Autodesk Inventor part; units mm, degrees
ref_plane "Work Plane2" through (7.15, 0, -16.233) normal (1, 0, 0) x (0, 0, -1)
ref_plane "Work Plane3" through (7.15, 0, -2.05) normal (1, 0, 0) x (0, 0, -1)
ref_plane "YZ Plane" through (0, 0, 0) normal (1, 0, 0) x (0, 1, 0)
sketch "Sketch1" plane through (0, 0, 0) normal (0, 1, 0) x (-1, 0, 0)
  line L0 (0, 0) -> (22.85, 0)
  line L1 (22.85, 0) -> (22.85, -100)
  line L2 (22.85, -100) -> (0, -100)
  line L3 (0, -100) -> (0, 0)
  circle A0 centre (7.12, -92.8) radius 4
  circle A1 centre (7.12, -64.4) radius 4
  circle A2 centre (7.12, -35.95) radius 4
  circle A3 centre (7.12, -7.71) radius 4
  circle A4 centre (7.12, -21.73) radius 1.5
  circle A5 centre (7.12, -49.67) radius 1.5
  circle A6 centre (7.12, -78.83) radius 1.5
  line L4 (7.12, -7.71) -> (-9.9799, -7.71) construction
  line L5 (7.12, -35.95) -> (-7.15, -35.95) construction
  line L6 (7.12, -64.4) -> (-7.15, -64.4) construction
  line L7 (7.12, -92.8) -> (-7.15, -92.8) construction
  line L8 (0, -27.427) -> (-7.15, -27.427)
  line L9 (0, -44.473) -> (-7.15, -44.473)
  line L10 (0, -55.877) -> (-7.15, -55.877)
  line L11 (0, -72.923) -> (-7.15, -72.923)
  line L12 (0, -84.277) -> (-7.15, -84.277)
  line L13 (0, -98.46) -> (-7.15, -98.46)
  line L14 (0, -2.05) -> (-7.15, -2.05)
  line L15 (0, -16.233) -> (-7.15, -16.233)
  line L16 (-7.15, -2.05) -> (-7.15, -16.233)
  line L17 (-7.15, -27.427) -> (-7.15, -44.473)
  line L18 (-7.15, -55.877) -> (-7.15, -72.923)
  line L19 (-7.15, -84.277) -> (-7.15, -98.46)
  line L20 (-7.15, 0) -> (-7.15, -100) construction
  dimension "d0" = 22.85
  dimension "d1" = 100
  dimension "d2" = 8
  dimension "d3" = 8
  dimension "d4" = 8
  dimension "d5" = 8
  dimension "d7" = 0
  dimension "d8" = 0
  dimension "d9" = 0
  dimension "d10" = 7.71
  dimension "d11" = 35.95
  dimension "d12" = 64.4
  dimension "d13" = 92.8
  dimension "d14" = 3
  dimension "d15" = 3
  dimension "d16" = 3
  dimension "d17" = 7.12
  dimension "d18" = 7.12
  dimension "d19" = 0
  dimension "d20" = 0
  dimension "d21" = 21.73
  dimension "d22" = 49.67
  dimension "d23" = 78.83
  dimension "d28" = 8.523
  dimension "d29" = 8.523
  dimension "d30" = 8.523
  dimension "d31" = 8.523
  dimension "d32" = 8.523
  dimension "d33" = 5.66
  dimension "d34" = 5.66
  dimension "d35" = 8.523
  dimension "d36" = 100
  dimension "d42" = 7.15
extrude "Extrusion1" add sketch "Sketch1" against normal blind 3
ref_plane "Work Plane2" through (7.15, 0, -16.233) normal (1, 0, 0) x (0, 0, -1)
ref_plane "Work Plane3" through (7.15, 0, -2.05) normal (1, 0, 0) x (0, 0, -1)
sketch "Sketch3" plane through (7.15, 0, -2.05) normal (1, 0, 0) x (0, 0, -1)
  line L0 (0, 0) -> (14.183, 0)
  line L1 (14.183, -3) -> (0, -3)
  line L2 (14.183, 0) -> (14.183, -3)
  line L3 (0, 0) -> (0, -3)
  line L4 (25.377, 0) -> (42.423, 0)
  line L5 (25.377, 0) -> (25.377, -3)
  line L6 (42.423, -3) -> (25.377, -3)
  line L7 (42.423, 0) -> (42.423, -3)
  line L8 (53.827, 0) -> (70.873, 0)
  line L9 (53.827, 0) -> (53.827, -3)
  line L10 (70.873, -3) -> (53.827, -3)
  line L11 (70.873, 0) -> (70.873, -3)
  line L12 (82.227, 0) -> (96.41, 0)
  line L13 (82.227, 0) -> (82.227, -3)
  line L14 (96.41, -3) -> (82.227, -3)
  line L15 (96.41, 0) -> (96.41, -3)
  line L16 (0, 0) -> (0, -40)
  line L17 (0, -40) -> (5.4, -40)
  line L18 (14.183, 0) -> (14.183, -20)
  line L19 (5.4, -40) -> (5.4, -28.783)
  line L20 (14.183, -20) -> (5.4, -28.783)
  line L21 (96.41, 0) -> (96.41, -40)
  line L22 (96.41, -40) -> (91.01, -40)
  line L23 (82.227, 0) -> (82.227, -20)
  line L24 (91.01, -40) -> (91.01, -28.783)
  line L25 (82.227, -20) -> (91.01, -28.783)
  line L26 (70.873, 0) -> (70.873, -20)
  line L27 (53.827, 0) -> (53.827, -20)
  line L28 (70.873, -20) -> (65.05, -25.823)
  line L29 (65.05, -25.823) -> (65.05, -40)
  line L30 (65.05, -40) -> (59.65, -40)
  line L31 (59.65, -40) -> (59.65, -25.823)
  line L32 (59.65, -25.823) -> (53.827, -20)
  line L33 (62.35, -40) -> (62.35, 0) construction
  line L34 (53.827, 0) -> (70.873, 0)
  line L35 (42.423, 0) -> (42.423, -20)
  line L36 (25.377, 0) -> (25.377, -20)
  line L37 (42.423, -20) -> (36.6, -25.823)
  line L38 (36.6, -25.823) -> (36.6, -40)
  line L39 (36.6, -40) -> (31.2, -40)
  line L40 (31.2, -40) -> (31.2, -25.823)
  line L41 (31.2, -25.823) -> (25.377, -20)
  line L42 (33.9, -40) -> (33.9, 0) construction
  point P0 (82.227, -3)
  dimension "d46" = 40
  dimension "d47" = 5.4
  dimension "d48" = 20
  dimension "d51" = 135
  dimension "d56" = 135
  dimension "d57" = 5.4
  dimension "d58" = 40
  dimension "d59" = 20
  dimension "d61" = 20
  dimension "d62" = 135
  dimension "d63" = 135
  dimension "d64" = 5.4
  dimension "d66" = 20
  dimension "d67" = 20
  dimension "d68" = 135
  dimension "d69" = 135
  dimension "d70" = 5.4
  dimension "d71" = 20
extrude "Extrusion2" add sketch "Sketch3" against normal blind 3
fillet "Fillet1" radius 4 4 edges at (7.15, 0, -9.1415) (7.15, 0, -35.95) (7.15, 0, -64.4) (7.15, 0, -91.3685)
chamfer "Chamfer1" distance 4 angle 45 4 edges at (4.15, -3, -9.1415) (4.15, -3, -35.95) (4.15, -3, -64.4) (4.15, -3, -91.3685)
equation "\"d18\" = d17"
equation "\"d57\" = d47"
equation "\"d58\" = d46"
equation "\"d59\" = d48"
properties part number "suporte 555"
CAD build for the part. Positions are in the model's coordinates, mm. A direction names the side the tool comes from. Round coordinates to 2 decimals unless told otherwise and drop trailing zeros. Loops run counter-clockwise (first coordinate to the right, second up) from the corner with the lowest first, then second, coordinate; pieces in that order, holes last. Notation, with made-up numbers: M 88,23 L 101,23 A29 cw 101,56 Z; hole C 32,12.25 d9. An arc over 180 degrees is marked long. Return JSON: item names as keys, results as strings. Group by question number.
(1) Drop flat-ended pins along their axis: P1, Ø1, axis at x = -18.5, z = -79.5, coming from the +Y side; P2, Ø1.5, axis at y = -1.5, z = -78, coming from the +X side; P3, Ø3, axis at x = 2, y = -28.5, coming from the -Z side; P4, Ø0.9, axis at x = 5, y = -37, coming from the -Z side. Give the stop position or say it passes through.
(2) Saw through at A-A, the plane z = -64.4. List the corners of the cut face in (x, y).
(3) Wall check: probe 1 along X at (y, z) = (-22.5, -11); probe 2 along X at (y, z) = (-2, -48.5); probe 3 along Y at (x, z) = (-21.5, -49). Give the ranges that are in metal, low to high. Write a range as [from, to].
(4) Saw through at B-B, the plane y = -34. List the corners of the cut face in (x, z), and give its area (3 significant figures).
(5) Saw through at D-D, the plane x = -7.12. Give the number of separate pieces and of enclosed holes in the cut face, and give its area (3 significant figures).
(6) Mould opens along Z. For faces 4 (the flat face through (4.15, -20, -7)), 5 (the cylindrical face through (-8.966, -1.479, -96.349)), 6 (the flat face through (5, -20, -98.46)) say: +Z half, -Z half, draft (parallel to the pull), parting line (faces both ways), or undercut.
(7) Saw through at C-C, the plane x = 2.25. List the corners of the cut face in (y, z), and give its area (3 significant figures).
(8) Tool access for faces 1 (the flat face through (6, -34, -93.06)), 2 (the flat face through (4.32, -7.64, -44.473)), 3 (the flat face through (4.15, -20, -93)): list every direction of +Z, -Z, +X, -X, +Y, -Y with a clear straight run to the whole face (end or side of a thin tool).
Answer list:
{
 "1": {"P1": "y = 0", "P2": "x = 0", "P3": "through", "P4": "z = -98.46"},
 "2": {"outline": "M -22.85,-3 L -11.12,-3 L -11.12,0 L -22.85,0 Z; M -3.12,-3 L 0.15,-3 L 4.15,-7 L 4.15,-40 L 7.15,-40 L 7.15,-4 A4 ccw 3.15,0 L -3.12,0 Z"},
 "3": {"probe 1": "[4.15, 7.15]", "probe 2": "[-22.85, -8.06], [-6.18, 0]", "probe 3": "[-3, 0]"},
 "4": {"outline": "M 4.15,-98.46 L 7.15,-98.46 L 7.15,-93.06 L 4.15,-93.06 Z; M 4.15,-67.1 L 7.15,-67.1 L 7.15,-61.7 L 4.15,-61.7 Z; M 4.15,-38.65 L 7.15,-38.65 L 7.15,-33.25 L 4.15,-33.25 Z; M 4.15,-7.45 L 7.15,-7.45 L 7.15,-2.05 L 4.15,-2.05 Z", "area": "64.8 mm2"},
 "5": {"separate pieces": "8", "enclosed holes": "0", "area": "177 mm2"},
 "6": {"face 4": "draft", "face 5": "undercut", "face 6": "-Z half"},
 "7": {"outline": "M -5.1,-98.46 L 0,-98.46 L 0,-84.28 L -5.1,-84.28 Z; M -5.1,-72.92 L 0,-72.92 L 0,-55.88 L -5.1,-55.88 Z; M -5.1,-44.47 L 0,-44.47 L 0,-27.43 L -5.1,-27.43 Z; M -5.1,-16.23 L 0,-16.23 L 0,-2.05 L -5.1,-2.05 Z", "area": "319 mm2"},
 "8": {"face 1": "+X, -X, -Y", "face 2": "+X, +Y, -Y", "face 3": "+Z, -Z, -X, -Y"}
}
